```python
from build123d import *

# Parameters (mm, degrees)
SKETCH1_W                                           = 336.55
SKETCH1_H                                           = 47.625
BOSS_EXTRUDE1_DEPTH                                 = 3.175
CSK_FOR_1_4_FLAT_HEAD_MACHINE_SCREW_100_D           = 6.7564
CSK_FOR_1_4_FLAT_HEAD_MACHINE_SCREW_100_CSINK_D     = 12.8778
CSK_FOR_1_4_FLAT_HEAD_MACHINE_SCREW_100_CSINK_ANGLE = 100
SKETCH4_W                                           = 10.998522628
SKETCH4_H                                           = 6.35
CUT_EXTRUDE1_DEPTH                                  = 1
CUT_EXTRUDE1_DEPTH_BACK                             = 337.55


with BuildPart() as part:
    # Sketch1 → Boss-Extrude1 (new body, symmetric)
    with BuildSketch(Plane(origin=(0, 0, 0), x_dir=(1, 0, 0), z_dir=(0, 1, 0))):
        Rectangle(SKETCH1_W, SKETCH1_H)
    extrude(amount=BOSS_EXTRUDE1_DEPTH, both=True)

    # CSK for 1/4 Flat Head Machine Screw (100)1 (through all)
    with Locations(Plane(origin=(0, 3.175, 0), x_dir=(1, 0, 0), z_dir=(0, 1, 0))):
        with Locations((-157.00375, 0), (157.00375, 0)):
            CounterSinkHole(CSK_FOR_1_4_FLAT_HEAD_MACHINE_SCREW_100_D / 2, CSK_FOR_1_4_FLAT_HEAD_MACHINE_SCREW_100_CSINK_D / 2, counter_sink_angle=CSK_FOR_1_4_FLAT_HEAD_MACHINE_SCREW_100_CSINK_ANGLE)

    # Sketch4 → Cut-Extrude1 (cut, two sides)
    with BuildSketch(Plane.ZY.offset(168.275)) as cut_extrude1_sk:
        with Locations((-18.313238686, 0)):
            Rectangle(SKETCH4_W, SKETCH4_H)
    extrude(amount=CUT_EXTRUDE1_DEPTH, mode=Mode.SUBTRACT)
    extrude(cut_extrude1_sk.sketch, amount=-CUT_EXTRUDE1_DEPTH_BACK, mode=Mode.SUBTRACT)


solid = part.part
```
Source: CAD feature listing. Evaluate the final solid. Frame: model axes, mm. Round coordinates to 2 decimals unless told otherwise and drop trailing zeros. Order: outer loops, then holes, each group sorted by start corner. A loop starts at its lowest first (then second) coordinate and runs counter-clockwise, first axis right, second up. Notation, with made-up numbers: (85.25, 78) -> (99.25, 78) arc R28 ccw to (99.25, 108) -> close; hole circle Ø1 at (44, 30.25). An arc over 180 degrees is marked (long way). Use CSV: the item, a comma, the result in double quotes.
(1) Section A-A on z = 0. Return the cut outline in (x, y) (3 decimals).
Report:
outline,"(-168.275, -3.175) -> (-160.382, -3.175) -> (-160.382, 0.607) -> (-163.443, 3.175) -> (-168.275, 3.175) -> close; (-153.626, -3.175) -> (153.626, -3.175) -> (153.626, 0.607) -> (150.565, 3.175) -> (-150.565, 3.175) -> (-153.626, 0.607) -> close; (160.382, -3.175) -> (168.275, -3.175) -> (168.275, 3.175) -> (163.443, 3.175) -> (160.382, 0.607) -> close"
(2) First-contact query: pin 1 Ø6 at (x, z) = (-157, 0) entering from -Y; pin 2 Ø8 at (x, z) = (157, 0) entering from +Y. Flat tips, straight axial feed; report the tip coordinate or a pass-through.
Report:
pin 1,"through"
pin 2,"y = 1.13"
(3) Pull-direction query (X, two-part tool) for faces 1 (the face through (-2, 0, -12.814)), 2 (the face through (-168.275, 0, 6)), 3 (the face through (-160.26, 0.73, 1.35)), 4 (the face through (153.78, -1.31, -1.01)); classes: +X half, -X half, draft (parallel to the pull), parting line (faces both ways), or undercut.
Report:
face 1,"draft"
face 2,"-X half"
face 3,"undercut"
face 4,"undercut"
(4) Ray query, L1, parallel to X at y = -0.5, z = -2.5 (3 decimals); L2, parallel to X at y = 1.75, z = 0.5 (3 decimals); L3, parallel to Z at x = 152.5, y = 2.5. Return the intervals inside material, ascending.
Report:
L1,"-168.275 to -159.276, -154.732 to 154.732, 159.276 to 168.275"
L2,"-168.275 to -161.718, -152.29 to 152.29, 161.718 to 168.275"
L3,"-12.81 to -3.39, 3.39 to 23.81"
